Geometry: final body of the model. Coordinates: model frame, mm. A direction names the side the tool comes from. Round coordinates to 2 decimals unless told otherwise and drop trailing zeros. Loops run counter-clockwise (first coordinate to the right, second up) from the corner with the lowest first, then second, coordinate; pieces in that order, holes last. Notation, with made-up numbers: M -10,25.25 L 16,25.25 A4 ccw 16,30.25 Z; hole C 12,76.5 d3. An arc over 180 degrees is marked long. Return JSON: item names as keys, results as strings.
from build123d import *

# Parameters (mm, degrees)
SKETCH1_W            = 26
SKETCH1_H            = 14.5
SKETCH1_W_2          = 24
SKETCH1_H_2          = 12.5
BOSS_EXTRUDE1_DEPTH  = 22
SKETCH2_W            = 3
SKETCH2_H            = 14.5
BOSS_EXTRUDE2_DEPTH  = 6
CUT_EXTRUDE1_REACH   = 40.823
SKETCH3_W            = 16
SKETCH3_H            = 12
CUT_EXTRUDE2_REACH   = 55.873
SKETCH4_R            = 1
SKETCH5_W            = 44
SKETCH5_H            = 44
SKETCH5_W_2          = 38.1
SKETCH5_H_2          = 38.1
BOSS_EXTRUDE3_DEPTH  = 40
SKETCH8_W            = 52
SKETCH8_H            = 52
SKETCH8_W_2          = 44
SKETCH8_H_2          = 44
BOSS_EXTRUDE5_DEPTH  = 36
SKETCH6_R            = 25
CUT_EXTRUDE5_DEPTH   = 2
BOSS_EXTRUDE6_DEPTH  = 4
CHAMFER1_SIZE        = 12
CUT_EXTRUDE7_REACH   = 83.884
SKETCH11_W           = 30
SKETCH11_H           = 28
CUT_EXTRUDE8_REACH   = 72.569
SKETCH12_W           = 30
SKETCH12_H           = 28
CHAMFER3_SIZE        = 4
SKETCH14_R           = 1.5
BOSS_EXTRUDE7_DEPTH  = 5
SKETCH15_W           = 38.1
SKETCH15_H           = 38.1
SKETCH15_W_2         = 33.1
SKETCH15_H_2         = 33.1
BOSS_EXTRUDE8_DEPTH  = 2
SKETCH16_W           = 15.4
SKETCH16_H           = 4
BOSS_EXTRUDE9_DEPTH  = 20
CUT_EXTRUDE10_START  = -44
SKETCH18_R           = 4.765
CUT_EXTRUDE10_DEPTH  = 44
FILLET4_RADIUS       = 7.7
FILLET4_LENGTH       = 4
FILLET5_RADIUS       = 7.7
FILLET5_LENGTH       = 4
BOSS_EXTRUDE10_REACH = 83.884
CUT_EXTRUDE12_REACH  = 70.389
SKETCH15_3_W         = 33.1
SKETCH15_3_H         = 33.1


# Some blends are built 0.0001 mm under size
with BuildPart() as part:
    # Sketch1 → Boss-Extrude1 (new body)
    with BuildSketch(Plane.XY):
        with Locations((12, 6.25)):
            Rectangle(SKETCH1_W, SKETCH1_H)
        with Locations((12, 6.25)):
            Rectangle(SKETCH1_W_2, SKETCH1_H_2, mode=Mode.SUBTRACT)
    boss_extrude1 = extrude(amount=BOSS_EXTRUDE1_DEPTH)

    # Sketch2 → Boss-Extrude2 (add)
    with BuildSketch(Plane.XY.offset(22)):
        with Locations((-2.5, 6.25)):
            Rectangle(SKETCH2_W, SKETCH2_H)
        with Locations((26.5, 6.25)):
            Rectangle(SKETCH2_W, SKETCH2_H)
    boss_extrude2 = extrude(amount=-BOSS_EXTRUDE2_DEPTH)

    # Mirror2: Boss-Extrude1, Boss-Extrude2 across plane
    add(boss_extrude1.mirror(Plane(origin=(0, 0, 0), x_dir=(1, 0, 0), z_dir=(0, 0, -1))))
    add(boss_extrude2.mirror(Plane(origin=(0, 0, 0), x_dir=(1, 0, 0), z_dir=(0, 0, -1))))

    # Cut-Extrude1: up to this face of the body (flat: up to its plane)
    cut_extrude1_end = Plane(part.part.faces().sort_by_distance((25, 6.25, 0))[0])
    # Sketch3 → Cut-Extrude1 (cut, up to the picked face)
    with BuildSketch(Plane.ZY.offset(1), mode=Mode.PRIVATE) as cut_extrude1_sk1:
        with Locations((0, 6.25)):
            Rectangle(SKETCH3_W, SKETCH3_H)
    cut_extrude1_tool1 = split(extrude(cut_extrude1_sk1.sketch, amount=-CUT_EXTRUDE1_REACH, mode=Mode.PRIVATE), bisect_by=cut_extrude1_end, keep=Keep.BOTH, mode=Mode.PRIVATE)
    add(cut_extrude1_tool1.solids().sort_by(Axis((-1, 6.25, 0), (1, 0, 0)))[0], mode=Mode.SUBTRACT)

    # Sketch4 → Cut-Extrude2 (cut, up to next)
    with BuildSketch(Plane.XY.offset(22), mode=Mode.PRIVATE) as cut_extrude2_sk1:
        with Locations((-1.59, 6.25)):
            Circle(SKETCH4_R)
    cut_extrude2_tool1 = extrude(cut_extrude2_sk1.sketch, amount=-CUT_EXTRUDE2_REACH, mode=Mode.PRIVATE) & part.part
    # Sketch4 → Cut-Extrude2 (cut, up to next)
    with BuildSketch(Plane.XY.offset(22), mode=Mode.PRIVATE) as cut_extrude2_sk2:
        with Locations(Location((25.59, 6.25, 0), (0, 0, 233.842991799))):
            Circle(SKETCH4_R)
    cut_extrude2_tool2 = extrude(cut_extrude2_sk2.sketch, amount=-CUT_EXTRUDE2_REACH, mode=Mode.PRIVATE) & part.part
    add(cut_extrude2_tool1.solids().sort_by_distance((-1.59, 6.25, 22))[0], mode=Mode.SUBTRACT)
    add(cut_extrude2_tool1.solids().sort_by_distance((-1.59, 6.25, 22))[1], mode=Mode.SUBTRACT)
    add(cut_extrude2_tool2.solids().sort_by_distance((25.59, 6.25, 22))[0], mode=Mode.SUBTRACT)
    add(cut_extrude2_tool2.solids().sort_by_distance((25.59, 6.25, 22))[1], mode=Mode.SUBTRACT)

    # Sketch5 → Boss-Extrude3 (add)
    with BuildSketch(Plane(origin=(0, 0, 0), x_dir=(0, 0, -1), z_dir=(1, 0, 0))):
        with Locations((0, -23)):
            Rectangle(SKETCH5_W, SKETCH5_H)
        with Locations((0, -23)):
            Rectangle(SKETCH5_W_2, SKETCH5_H_2, mode=Mode.SUBTRACT)
    extrude(amount=-BOSS_EXTRUDE3_DEPTH)

    # Sketch8 → Boss-Extrude5 (add)
    with BuildSketch(Plane.ZY.offset(40)):
        with Locations((0, -23)):
            Rectangle(SKETCH8_W, SKETCH8_H)
        with Locations((0, -23)):
            Rectangle(SKETCH8_W_2, SKETCH8_H_2, mode=Mode.SUBTRACT)
    extrude(amount=-BOSS_EXTRUDE5_DEPTH)

    # Sketch6 → Cut-Extrude5 (cut)
    with BuildSketch(Plane.ZY.offset(40)):
        with Locations((0, -23)):
            Circle(SKETCH6_R)
    extrude(amount=-CUT_EXTRUDE5_DEPTH, mode=Mode.SUBTRACT)

    # Sketch9 → Boss-Extrude6 (add)
    with BuildSketch(Plane(origin=(-4, 0, 0), x_dir=(0, 0, -1), z_dir=(1, 0, 0))):
        Polygon((-26, -49), (26, -49), (26, -1), (22, -1), (22, -45), (-22, -45), (-22, -1), (-26, -1), align=None)
    extrude(amount=BOSS_EXTRUDE6_DEPTH)

    # Chamfer1
    # the kernel refuses this chamfer: 12 mm, written as the material it takes off along each edge
    with BuildSketch(Plane(origin=(-70.860195856, 3, 26), x_dir=(0, 0.027495876610586382, -0.9996219169112968), z_dir=(1, 0, 0))) as chamfer1_piece_1:
        Polygon((CHAMFER1_SIZE * 0.999621916911, -CHAMFER1_SIZE * 0.0274958766106), (-CHAMFER1_SIZE * 0.0274958766106, -CHAMFER1_SIZE * 0.999621916911), (0, 0), align=None)
    extrude(amount=66.860195856, mode=Mode.SUBTRACT)
    with BuildSketch(Plane(origin=(30.860195856, -49, 26), x_dir=(0, -0.027495876610586202, -0.9996219169112968), z_dir=(-1, 0, 0)), Plane(origin=(-70.860195856, -49, -26), x_dir=(0, -0.027495876610586202, 0.9996219169112968), z_dir=(1, 0, 0))) as chamfer1_piece_2:
        Polygon((CHAMFER1_SIZE * 0.999621916911, -CHAMFER1_SIZE * 0.0274958766106), (-CHAMFER1_SIZE * 0.0274958766106, -CHAMFER1_SIZE * 0.999621916911), (0, 0), align=None)
    extrude(amount=101.720391711, mode=Mode.SUBTRACT)
    with BuildSketch(Plane(origin=(-70.860195856, 3, -26), x_dir=(0, 0.027495876610586382, 0.9996219169112968), z_dir=(1, 0, 0))) as chamfer1_piece_3:
        Polygon((CHAMFER1_SIZE * 0.999621916911, CHAMFER1_SIZE * 0.0274958766106), (-CHAMFER1_SIZE * 0.0274958766106, CHAMFER1_SIZE * 0.999621916911), (0, 0), align=None)
    extrude(amount=66.860195856, mode=Mode.SUBTRACT)

    # Cut-Extrude7: up to this face of the body (flat: up to its plane)
    cut_extrude7_end = Plane(part.part.faces().sort_by_distance((-19.5, -22.5, -26))[0])
    # Sketch11 → Cut-Extrude7 (cut, up to the picked face)
    with BuildSketch(Plane.XY.offset(26), mode=Mode.PRIVATE) as cut_extrude7_sk1:
        with Locations((-20, -23)):
            Rectangle(SKETCH11_W, SKETCH11_H)
    cut_extrude7_tool1 = split(extrude(cut_extrude7_sk1.sketch, amount=-CUT_EXTRUDE7_REACH, mode=Mode.PRIVATE), bisect_by=cut_extrude7_end, keep=Keep.BOTH, mode=Mode.PRIVATE)
    add(cut_extrude7_tool1.solids().sort_by(Axis((-20, -23, 26), (0, 0, -1)))[0], mode=Mode.SUBTRACT)

    # Cut-Extrude8: up to this face of the body (flat: up to its plane)
    cut_extrude8_end = Plane(part.part.faces().sort_by_distance((-20, -49, 0))[0])
    # Sketch12 → Cut-Extrude8 (cut, up to the picked face)
    with BuildSketch(Plane(origin=(0, 3, 0), x_dir=(1, 0, 0), z_dir=(0, 1, 0)), mode=Mode.PRIVATE) as cut_extrude8_sk1:
        with Locations((-20, 0)):
            Rectangle(SKETCH12_W, SKETCH12_H)
    cut_extrude8_tool1 = split(extrude(cut_extrude8_sk1.sketch, amount=-CUT_EXTRUDE8_REACH, mode=Mode.PRIVATE), bisect_by=cut_extrude8_end, keep=Keep.BOTH, mode=Mode.PRIVATE)
    add(cut_extrude8_tool1.solids().sort_by(Axis((-20, 3, 0), (0, -1, 0)))[0], mode=Mode.SUBTRACT)

    # Chamfer3
    chamfer3_edges = [part.edges().sort_by_distance(p)[0] for p in [
        (-2, -1, -26),
        (-2, -1, 26),
    ]]
    chamfer(chamfer3_edges, length=CHAMFER3_SIZE - 0.0001)  # a hair under: the kernel refuses the full size

    # Sketch14 → Boss-Extrude7 (add)
    # profile 1 of 4: a face of its own
    with BuildSketch(Plane.ZY.offset(40)):
        Polygon((-26, 3), (-14, 3), (-26, -9), align=None)
        with Locations((-23, 0)):
            Circle(SKETCH14_R, mode=Mode.SUBTRACT)
    # profile 2 of 4: a face of its own
    with BuildSketch(Plane.ZY.offset(40)):
        Polygon((14, 3), (26, -9), (26, 3), align=None)
        with Locations((23, 0)):
            Circle(SKETCH14_R, mode=Mode.SUBTRACT)
    # profile 3 of 4: a face of its own
    with BuildSketch(Plane.ZY.offset(40)):
        Polygon((26, -49), (14, -49), (26, -37), align=None)
        with Locations((23, -46)):
            Circle(SKETCH14_R, mode=Mode.SUBTRACT)
    # profile 4 of 4: a face of its own
    with BuildSketch(Plane.ZY.offset(40)):
        Polygon((-26, -49), (-26, -37), (-14, -49), align=None)
        with Locations((-23, -46)):
            Circle(SKETCH14_R, mode=Mode.SUBTRACT)
    extrude(amount=-BOSS_EXTRUDE7_DEPTH)

    # Sketch15 → Boss-Extrude8 (add)
    with BuildSketch(Plane(origin=(0, 0, 0), x_dir=(0, 0, -1), z_dir=(1, 0, 0))):
        with Locations((0, -23)):
            Rectangle(SKETCH15_W, SKETCH15_H)
        with Locations((0, -23)):
            Rectangle(SKETCH15_W_2, SKETCH15_H_2, mode=Mode.SUBTRACT)
    extrude(amount=-BOSS_EXTRUDE8_DEPTH)

    # Sketch16 → Boss-Extrude9 (add)
    with BuildSketch(Plane(origin=(0, 13.5, 0), x_dir=(1, 0, 0), z_dir=(0, 1, 0))):
        with Locations((17.3, -20)):
            Rectangle(SKETCH16_W, SKETCH16_H)
        with Locations((17.3, 20)):
            Rectangle(SKETCH16_W, SKETCH16_H)
    extrude(amount=BOSS_EXTRUDE9_DEPTH)

    # Sketch18 → Cut-Extrude10 (cut)
    with BuildSketch(Plane.XY.offset(22).offset(CUT_EXTRUDE10_START)):
        with Locations((17.3, 25.5)):
            Circle(SKETCH18_R)
    extrude(amount=CUT_EXTRUDE10_DEPTH, mode=Mode.SUBTRACT)

    # Fillet4: full round fillet: the end face becomes a half cylinder, R = half its width
    fillet4_face = Plane((17.3, 33.5, 20), x_dir=(0, 0, -1), z_dir=(0, 1, 0))  # on the end face: x along it, z out of the body
    fillet4_slab = fillet4_face.offset(-FILLET4_RADIUS / 2) * Box(FILLET4_LENGTH, 2 * FILLET4_RADIUS, FILLET4_RADIUS, mode=Mode.PRIVATE)  # the body's end, R deep
    fillet4_round = Plane((17.3, 25.8, 20), x_dir=(0, 1, 0), z_dir=(0, 0, -1)) * Cylinder(FILLET4_RADIUS, FILLET4_LENGTH, mode=Mode.PRIVATE)  # its axis R under the face
    add(fillet4_slab - fillet4_round, mode=Mode.SUBTRACT)

    # Fillet5: full round fillet: the end face becomes a half cylinder, R = half its width
    fillet5_face = Plane((17.3, 33.5, -20), x_dir=(0, 0, -1), z_dir=(0, 1, 0))  # on the end face: x along it, z out of the body
    fillet5_slab = fillet5_face.offset(-FILLET5_RADIUS / 2) * Box(FILLET5_LENGTH, 2 * FILLET5_RADIUS, FILLET5_RADIUS, mode=Mode.PRIVATE)  # the body's end, R deep
    fillet5_round = Plane((17.3, 25.8, -20), x_dir=(0, 1, 0), z_dir=(0, 0, -1)) * Cylinder(FILLET5_RADIUS, FILLET5_LENGTH, mode=Mode.PRIVATE)  # its axis R under the face
    add(fillet5_slab - fillet5_round, mode=Mode.SUBTRACT)

    # Boss-Extrude10: up to this face of the body (flat: up to its plane)
    boss_extrude10_end = Plane(part.part.faces().sort_by_distance((-2.448716798, -21.358932413, -26))[0])
    # Sketch19 → Boss-Extrude10 (add, up to the picked face)
    with BuildSketch(Plane.XY.offset(26), mode=Mode.PRIVATE) as boss_extrude10_sk1:
        Polygon((0, -49), (28, -1), (0, -1), align=None)
    boss_extrude10_tool1 = split(extrude(boss_extrude10_sk1.sketch, amount=-BOSS_EXTRUDE10_REACH, mode=Mode.PRIVATE), bisect_by=boss_extrude10_end, keep=Keep.BOTH, mode=Mode.PRIVATE)
    add(boss_extrude10_tool1.solids().sort_by(Axis((9.333333, -17, 26), (0, 0, -1)))[0])

    # Cut-Extrude12: up to this face of the body (flat: up to its plane)
    cut_extrude12_end = Plane(part.part.faces().sort_by_distance((14, -25, 0))[0])
    # Sketch15<3> → Cut-Extrude12 (cut, up to the picked face)
    with BuildSketch(Plane(origin=(0, 0, 0), x_dir=(0, 0, -1), z_dir=(1, 0, 0)), mode=Mode.PRIVATE) as cut_extrude12_sk1:
        with Locations((0, -23)):
            Rectangle(SKETCH15_3_W, SKETCH15_3_H)
    cut_extrude12_tool1 = split(extrude(cut_extrude12_sk1.sketch, amount=CUT_EXTRUDE12_REACH, mode=Mode.PRIVATE), bisect_by=cut_extrude12_end, keep=Keep.BOTH, mode=Mode.PRIVATE)
    add(cut_extrude12_tool1.solids().sort_by(Axis((0, -23, 0), (1, 0, 0)))[0], mode=Mode.SUBTRACT)


solid = part.part
Q1. Pull-direction query (Y, two-part tool) for faces 5 (the flat face through (-38, -49, 0)), 6 (the flat face through (0, 6, 10)), 7 (the flat face through (0, -2.5, 24.5)); classes: pulls with the +Y half, pulls with the -Y half, needs draft (parallel to the pull), parting line crosses it, or undercut.
Determined:
{"face 5": "pulls with the -Y half", "face 6": "undercut", "face 7": "needs draft"}
Q2. Material intervals for L1, parallel to X at y = 6.25, z = 18; L2, parallel to Y at x = -36, z = -23; L3, parallel to X at y = 25.5, z = 18.85 (3 decimals), sorted ascending.
Determined:
{"L1": "x = -4 to -2.59, -0.59 to 0, 24 to 24.59, 26.59 to 28", "L2": "y = -49 to -47.5, -44.5 to -1.5, 1.5 to 3", "L3": "x = 9.6 to 12.535, 22.065 to 25"}
Q3. Section query D-D (y = 16.5). Output: boundary loops of the cut face in (x, z).
Determined:
{"outline": "M 9.6,-22 L 25,-22 L 25,-18 L 9.6,-18 Z; M 9.6,18 L 25,18 L 25,22 L 9.6,22 Z"}
Q4. Pin query (flat end, axial travel): pin 1 (14 mm diameter, centred on y = 7, z = -6, fed in from +X); pin 2 (8 mm diameter, centred on x = -10.5, z = -9, fed in from -Y); pin 3 (3.5 mm diameter, centred on x = -24.5, z = 23.5, fed in from -Y); pin 4 (2 mm diameter, centred on x = -15.5, y = -38.5, fed in from -Z). Return the tip coordinate at first contact, or that it passes through.
Determined:
{"pin 1": "stops at x = 25", "pin 2": "passes through", "pin 3": "stops at y = -41.25", "pin 4": "stops at z = -25.5"}
Q5. Section query B-B (z = -23). State how many separate pieces and enclosed holes the cut face has, plus the area to 3 significant figures.
Determined:
{"separate pieces": "3", "enclosed holes": "1", "area": "1,230 mm^2"}
Q6. Section query A-A (x = -26). Output: boundary loops of the cut face in (y, z), plus the area to 3 significant figures.
Determined:
{"outline": "M -49,-14 L -37,-26 L -37,-19.05 L -42.05,-19.05 L -42.05,-14 Z; M -49,14 L -42.05,14 L -42.05,19.05 L -37,19.05 L -37,26 Z; M -9,-26 L 3,-14 L -3.95,-14 L -3.95,-19.05 L -9,-19.05 Z; M -9,19.05 L -3.95,19.05 L -3.95,14 L 3,14 L -9,26 Z", "area": "186 mm^2"}
Q7. Reachability of faces 1 (the flat face through (-35, -46, 21)), 2 (the flat face through (-5, -45, 0)), 3 (the flat face through (-2, -3, -24)), 4 (the flat face through (-20, -3, 20)) from +Z, -Z, +X, -X, +Y, -Y: full face, straight path, thin tool, end or side. Return the list, or none.
Determined:
{"face 1": "+Z, -Y", "face 2": "+Y, -Y", "face 3": "-Z, +Y", "face 4": "+Z, +Y"}
Q8. Section query C-C (y = -46). Output: boundary loops of the cut face in (x, z), plus the area to 3 significant figures.
Determined:
{"outline": "M -40,-26 L -35,-26 L -35,-24.5 L -40,-24.5 Z; M -40,-21.5 L -35,-21.5 L -35,-17 L 0,-17 L 0,-26 L 1.75,-26 L 1.75,26 L 0,26 L 0,17 L -35,17 L -35,21.5 L -40,21.5 L -40,9.8 L -38,9.8 L -38,-9.8 L -40,-9.8 Z; M -40,24.5 L -35,24.5 L -35,26 L -40,26 Z; hole M -35,-14 L -5,-14 L -5,14 L -35,14 Z", "area": "632 mm^2"}
